Source: CAD feature listing. Evaluate the final solid. Frame: model axes, mm. Face numbers are marked on the shaded views. A direction names the side the tool comes from. Give positions to 0.01 mm unless a question says otherwise; leave off trailing zeros. Loops run counter-clockwise (first coordinate to the right, second up) from the corner with the lowest first, then second, coordinate; pieces in that order, holes last.
from build123d import *

# Parameters (mm, degrees)
F0_R     = 24.014972
F1_DEPTH = 30.734
F2_R     = 11.066497
F3_DEPTH = 58.928
F4_W     = 10.073201
F4_H     = 9.49759
F5_DEPTH = 73.152
F6_W     = 10.073201
F6_H     = 4.029282
F7_DEPTH = 31.496


with BuildPart() as f1:
    # F0 (on Front) → F1 (new body)
    with BuildSketch(Plane.XZ):
        Circle(F0_R)
    extrude(amount=F1_DEPTH)

    # F2 (on Front) → F3 (join)
    with BuildSketch(Plane.XZ):
        Circle(F2_R)
    extrude(amount=F3_DEPTH)

    # F4 (on Front) → F5 (join)
    with BuildSketch(Plane.XZ):
        with Locations((1e-06, 0)):
            Rectangle(F4_W, F4_H)
    extrude(amount=F5_DEPTH)

    # F6 (on Top) → F7 (join)
    with BuildSketch(Plane.XY):
        with Locations((-0.287809, -70.656318)):
            Rectangle(F6_W, F6_H)
    extrude(amount=F7_DEPTH)


solid = f1.part
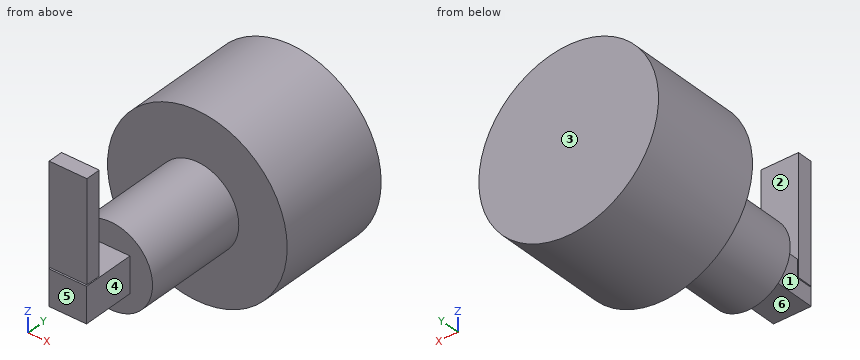
1) Cut plane B-B (z = 22.5). Return loops of the section in (x, y).
Checks:
outline: (-8.39, -30.73) - (8.39, -30.73) - (8.39, 0) - (-8.39, 0) - close; (-5.32, -72.67) - (4.75, -72.67) - (4.75, -68.64) - (-5.32, -68.64) - close
2) Cut plane A-A (x = 0). Return loops of the section in (y, z).
Checks:
outline: (-73.15, -4.75) - (-58.93, -4.75) - (-58.93, -11.07) - (-30.73, -11.07) - (-30.73, -24.01) - (0, -24.01) - (0, 24.01) - (-30.73, 24.01) - (-30.73, 11.07) - (-58.93, 11.07) - (-58.93, 4.75) - (-68.64, 4.75) - (-68.64, 31.5) - (-72.67, 31.5) - (-72.67, 4.75) - (-73.15, 4.75) - close
3) Contact query for flat-ended pins moving along their axis: P1, Ø1, axis at x = 14, z = 3.5, coming from the -Y side; P2, Ø8, axis at y = -59.5, z = 12, coming from the +X side; P3, Ø7.5, axis at y = -66, z = 2, coming from the +X side. Output: stop coordinate, or through.
Checks:
P1: stops at y = -30.73
P2: stops at x = 7.6
P3: stops at x = 5.04
4) Ray query, probe 1 along Y at (x, z) = (-5, 7.5); probe 2 along Y at (x, z) = (-4, 17); probe 3 along Y at (x, z) = (13.5, 17.5). Return the intervals inside material, ascending.
Checks:
probe 1: y = -72.67 to -68.64, -58.93 to 0
probe 2: y = -72.67 to -68.64, -30.73 to 0
probe 3: y = -30.73 to 0
5) Reachability of the marked faces 5 and 6 from +Z, -Z, +X, -X, +Y, -Y: full face, straight path, thin tool, end or side. Return the list, or none.
Checks:
face 5: +Z, -Z, +X, -X, -Y
face 6: -Z, +X, -X, -Y
6) Pull-direction query (Y, two-part tool) for the marked faces 1, 2, 3 and 4; classes: released by +Y, released by -Y, zero draft, split by the parting line, or undercut.
Checks:
face 1: undercut
face 2: undercut
face 3: released by +Y
face 4: zero draft
7) Cut plane C-C (y = -57.5). Return loops of the section in (x, z), and give its area (3 significant figures).
Checks:
outline: circle Ø22.13 at (0, 0)
area: 385 mm2
8) Cut plane D-D (z = 2.5). Return loops of the section in (x, y), and give its area (3 significant figures).
Checks:
outline: (-23.88, -30.73) - (-10.78, -30.73) - (-10.78, -58.93) - (-5.04, -58.93) - (-5.04, -68.64) - (-5.32, -68.64) - (-5.32, -72.67) - (-5.04, -72.67) - (-5.04, -73.15) - (5.04, -73.15) - (5.04, -58.93) - (10.78, -58.93) - (10.78, -30.73) - (23.88, -30.73) - (23.88, 0) - (-23.88, 0) - close
area: 2,220 mm2
